Design review of the part built by this model. Coordinates are the model's own, in mm. Give positions to 0.01 mm unless a question says otherwise; leave off trailing zeros. Loops run counter-clockwise (first coordinate to the right, second up) from the corner with the lowest first, then second, coordinate; pieces in that order, holes last. Notation, with made-up numbers: (54.5, 70.25) - (76.5, 70.25) arc R18 cw to (76.5, 88.25) - close; hole circle Ø6 at (-13, 4). An arc over 180 degrees is marked (long way). One line per item, written item: value. Start each with the question number.
```python
from build123d import *

# Parameters (mm, degrees)
F0_R     = 2.5
F1_DEPTH = 1


with BuildPart() as f1:
    # F0 (on Front) → F1 (new body)
    with BuildSketch(Plane.XZ):
        with BuildLine():
            ThreePointArc((-5, 37.5031), (0, 32.5031), (5, 37.5031))
            ThreePointArc((5, 37.5031), (0, 42.5031), (-5, 37.5031))
        make_face()
        with Locations((0, 37.5031)):
            Circle(F0_R, mode=Mode.SUBTRACT)
        with BuildLine():
            Line((5, -37.5031), (5, 37.5031))
            ThreePointArc((5, 37.5031), (0, 32.5031), (-5, 37.5031))
            Line((-5, 37.5031), (-5, -37.5031))
            ThreePointArc((-5, -37.5031), (0, -32.5031), (5, -37.5031))
        make_face()
        with Locations((0, 12.4969)):
            Circle(F0_R, mode=Mode.SUBTRACT)
        with BuildLine():
            ThreePointArc((-5, -37.5031), (0, -42.5031), (5, -37.5031))
            ThreePointArc((5, -37.5031), (0, -32.5031), (-5, -37.5031))
        make_face()
        with Locations((0, -37.5031)):
            Circle(F0_R, mode=Mode.SUBTRACT)
    extrude(amount=F1_DEPTH)


solid = f1.part
```
(1) Take a section at C-C on x = 4. State the section outline as (y, z) points, and give its area (3 significant figures).
(2) Draft analysis for pull direction Z (two halves, no side actions). For faces 1 (the flat face through (0, 0, 1)), 2 (the cylindrical face through (-0.325, -0.493, -35.024)), 3 (the cylindrical face through (0.11, -0.49, 42.5)), state which applies: pulls with the +Z half, pulls with the -Z half, needs draft (parallel to the pull), parting line crosses it, or undercut.
(3) To check wall thickness, follow L1, parallel to Z at x = 0, y = -0.8; L2, parallel to X at y = -0.3, z = 37.5; L3, parallel to X at y = -0.15, z = 38.5. State the ranges of each line that lie inside material, in increasing order. Write a range as from..to.
(4) Take a section at B-B on y = -0.35. State the section outline as (x, z) points.
(5) Take a section at A-A on x = 0. State the section outline as (y, z) points.
Here are the results:
1. outline: (-1, -40.5) - (0, -40.5) - (0, 40.5) - (-1, 40.5) - close
1. area: 81.0 mm²
2. face 1: needs draft
2. face 2: undercut
2. face 3: pulls with the +Z half
3. L1: -42.5..-40, -35..10, 15..35, 40..42.5
3. L2: -5..-2.5, 2.5..5
3. L3: -4.9..-2.29, 2.29..4.9
4. outline: (-5, -37.5) arc R5 ccw to (5, -37.5) - (5, 37.5) arc R5 ccw to (-5, 37.5) - close; hole circle Ø5 at (0, -37.5); hole circle Ø5 at (0, 12.5); hole circle Ø5 at (0, 37.5)
5. outline: (-1, -42.5) - (0, -42.5) - (0, -40) - (-1, -40) - close; (-1, -35) - (0, -35) - (0, 10) - (-1, 10) - close; (-1, 15) - (0, 15) - (0, 35) - (-1, 35) - close; (-1, 40) - (0, 40) - (0, 42.5) - (-1, 42.5) - close
